```python
from build123d import *

# Parameters (mm, degrees)
SKETCH1_W           = 4
SKETCH1_H           = 8
SKETCH1_H_2         = 4
BOSS_EXTRUDE1_DEPTH = 4


with BuildPart() as part:
    # Sketch1 → Boss-Extrude1 (new body)
    with BuildSketch(Plane(origin=(0, 0, 0), x_dir=(1, 0, 0), z_dir=(0, 1, 0))):
        with BuildLine():
            ThreePointArc((25, 31.224989992), (0, 40), (-25, 31.224989992))
            Line((-25, 31.224989992), (-25, -31.224989992))
            ThreePointArc((-25, -31.224989992), (0, -40), (25, -31.224989992))
            Line((25, -31.224989992), (25, 31.224989992))
        make_face()
        with Locations((-15, -30)):
            Rectangle(SKETCH1_W, SKETCH1_H, mode=Mode.SUBTRACT)
        with Locations((15, -30)):
            Rectangle(SKETCH1_W, SKETCH1_H, mode=Mode.SUBTRACT)
        with Locations((-20, 0)):
            Rectangle(SKETCH1_W, SKETCH1_H_2, mode=Mode.SUBTRACT)
        with Locations((-15, 30)):
            Rectangle(SKETCH1_W, SKETCH1_H, mode=Mode.SUBTRACT)
        with Locations((20, 0)):
            Rectangle(SKETCH1_W, SKETCH1_H_2, mode=Mode.SUBTRACT)
        with Locations((15, 30)):
            Rectangle(SKETCH1_W, SKETCH1_H, mode=Mode.SUBTRACT)
    extrude(amount=BOSS_EXTRUDE1_DEPTH)


solid = part.part
```
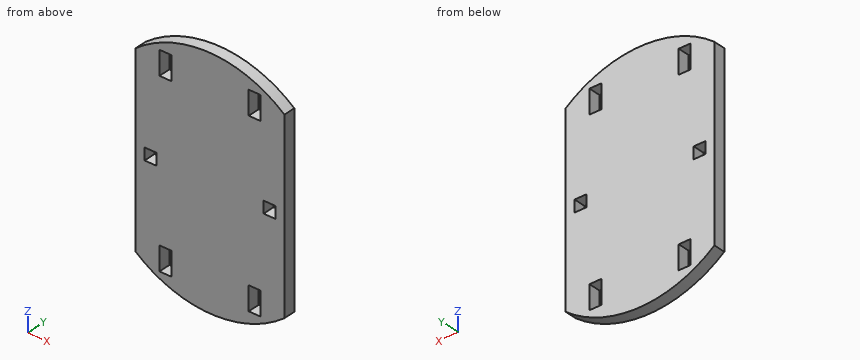
Geometry: final body of the model. Coordinates: model frame, mm. Coordinates: 2 decimals unless noted, no trailing zeros. Order: outer loops, then holes, each group sorted by start corner. A loop starts at its lowest first (then second) coordinate and runs counter-clockwise, first axis right, second up. Notation, with made-up numbers: (-23, 88) -> (21, 88) arc R35 ccw to (21, 121) -> close; hole circle Ø2 at (7.25, -10.5). An arc over 180 degrees is marked (long way). Write each question's results on one line, items separated by ' | '. Start each with the question number.
1) Cut plane D-D, the plane x = -19.5. Output: boundary loops of the cut face in (y, z).
2) First-contact query: pin 1 (1 mm diameter, centred on x = -15.5, y = 0.5, fed in from +Z); pin 2 (2 mm diameter, centred on x = -14.5, y = 2.5, fed in from +Z); pin 3 (2 mm diameter, centred on x = 12.5, y = 0.5, fed in from -Z). Flat tips, straight axial feed; report the tip coordinate or a pass-through.
3) Material intervals for line 1 along X through (y, z) = (3.45, 1.5); line 2 along X through (y, z) = (3.7, 30); line 3 along Z through (x, y) = (14, 1.5), sorted ascending.
4) Cut plane B-B, the plane y = 2.1. Output: boundary loops of the cut face in (x, z), and give its area (3 significant figures).
5) Cut plane A-A, the plane z = -27.5. Output: boundary loops of the cut face in (x, y), and give its area (3 significant figures).
6) Cut plane C-C, the plane x = 14. Output: boundary loops of the cut face in (y, z), and give its area (3 significant figures).
Checks:
1) outline: (0, -34.92) -> (4, -34.92) -> (4, -2) -> (0, -2) -> close; (0, 2) -> (4, 2) -> (4, 34.92) -> (0, 34.92) -> close
2) pin 1: z = 37.08 | pin 2: z = 37.65 | pin 3: z = -38.31
3) line 1: -25 to -22, -18 to 18, 22 to 25 | line 2: -25 to -17, -13 to 13, 17 to 25 | line 3: -37.47 to -34, -26 to 26, 34 to 37.47
4) outline: (-25, -31.22) arc R40 ccw to (25, -31.22) -> (25, 31.22) arc R40 ccw to (-25, 31.22) -> close; hole (-22, -2) -> (-18, -2) -> (-18, 2) -> (-22, 2) -> close; hole (-17, -34) -> (-13, -34) -> (-13, -26) -> (-17, -26) -> close; hole (-17, 26) -> (-13, 26) -> (-13, 34) -> (-17, 34) -> close; hole (13, -34) -> (17, -34) -> (17, -26) -> (13, -26) -> close; hole (13, 26) -> (17, 26) -> (17, 34) -> (13, 34) -> close; hole (18, -2) -> (22, -2) -> (22, 2) -> (18, 2) -> close | area: 3,560 mm^2
5) outline: (-25, 0) -> (-17, 0) -> (-17, 4) -> (-25, 4) -> close; (-13, 0) -> (13, 0) -> (13, 4) -> (-13, 4) -> close; (17, 0) -> (25, 0) -> (25, 4) -> (17, 4) -> close | area: 168 mm^2
6) outline: (0, -37.47) -> (4, -37.47) -> (4, -34) -> (0, -34) -> close; (0, -26) -> (4, -26) -> (4, 26) -> (0, 26) -> close; (0, 34) -> (4, 34) -> (4, 37.47) -> (0, 37.47) -> close | area: 236 mm^2
